from build123d import *

# Parameters (mm, degrees)
F0_W           = 47.661982
F0_H           = 44.654008
F1_DEPTH       = 25
F3_D           = 5
F3_CBORE_D     = 10
F3_CBORE_DEPTH = 5


with BuildPart() as f1:
    # F0 (on Front) → F1 (new body)
    with BuildSketch(Plane.XZ):
        with Locations((23.830991, 22.327004)):
            Rectangle(F0_W, F0_H)
    extrude(amount=F1_DEPTH)

    # F3 (through all)
    with Locations(Plane.XZ.offset(25)):
        with Locations((33.997253, 31.13661)):
            CounterBoreHole(F3_D / 2, F3_CBORE_D / 2, F3_CBORE_DEPTH)


solid = f1.part
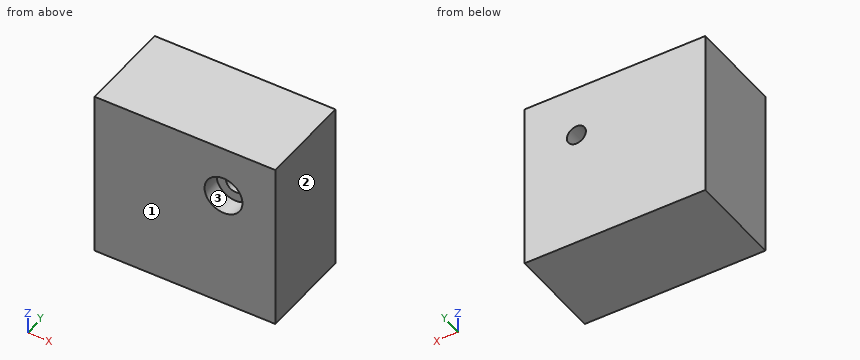
Geometry: final body of the model. Coordinates: model frame, mm. Face numbers are marked on the shaded views. Round coordinates to 2 decimals unless told otherwise and drop trailing zeros. Loops run counter-clockwise (first coordinate to the right, second up) from the corner with the lowest first, then second, coordinate; pieces in that order, holes last. Notation, with made-up numbers: M 88.5,74 L 96.5,74 A32 cw 96.5,112 Z; hole C -24,-37 d7. An arc over 180 degrees is marked long. Put each result on its own line as item: value. Start each with the question number.
(1) Contact query for a flat-ended pin moving along its axis: pin 1 Ø3 at (x, z) = (32, 31) entering from -Y. Output: stop coordinate, or through.
(2) Material intervals for line 1 along Y through (x, z) = (37.5, 32); line 2 along Z through (x, y) = (35, -6), sorted ascending. Write a range as [from, to].
(3) Section query A-A (x = 34). Return loops of the section in (y, z).
(4) Draft query along X for the marked faces 1, 2 and 3. Return one class per face: +X half, -X half, draft (parallel to the pull), parting line (faces both ways), or undercut.
(5) Section query C-C (y = -21). Return loops of the section in (x, z).
(6) Section query B-B (z = 30). Return loops of the section in (x, y).
Findings below:
1. pin 1: stops at y = -20
2. line 1: y = [-20, 0]
2. line 2: z = [0, 28.85], [33.43, 44.65]
3. outline: M -25,0 L 0,0 L 0,28.64 L -20,28.64 L -20,26.14 L -25,26.14 Z; M -25,36.14 L -20,36.14 L -20,33.64 L 0,33.64 L 0,44.65 L -25,44.65 Z
4. face 1: draft
4. face 2: +X half
4. face 3: undercut
5. outline: M 0,0 L 47.66,0 L 47.66,44.65 L 0,44.65 Z; hole C 34,31.14 d10
6. outline: M 0,-25 L 29.13,-25 L 29.13,-20 L 31.77,-20 L 31.77,0 L 0,0 Z; M 36.22,-20 L 38.87,-20 L 38.87,-25 L 47.66,-25 L 47.66,0 L 36.22,0 Z
